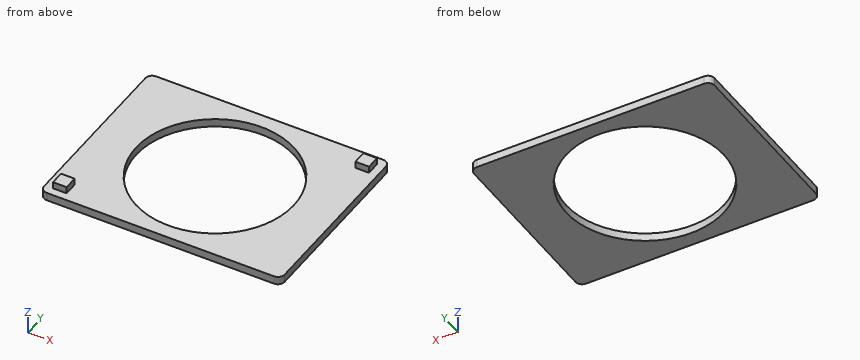
```python
from build123d import *

# Parameters (mm, degrees)
SKETCH007_W        = 35.4
SKETCH007_H        = 27.4
PAD002_DEPTH       = 1.2
FILLET001_R        = 1
SKETCH008_R        = 11.6
POCKET003_DEPTH    = 1.201
SKETCH009_W        = 2
SKETCH009_H        = 2
PAD003_DEPTH       = 1
POLARPATTERN_COUNT = 2


with BuildPart() as part:
    # Sketch007 → Pad002 (new body)
    with BuildSketch(Plane.XY):
        Rectangle(SKETCH007_W, SKETCH007_H)
    extrude(amount=PAD002_DEPTH)

    # Fillet001
    fillet001_edges = [part.edges().sort_by_distance(p)[0] for p in [
        (-17.7, -13.7, 0.6),
        (17.7, -13.7, 0.6),
        (17.7, 13.7, 0.6),
        (-17.7, 13.7, 0.6),
    ]]
    fillet(fillet001_edges, radius=FILLET001_R)

    # Sketch008 (on Face5 of Fillet001) → Pocket003 (cut, through all)
    with BuildSketch(Plane.XY.offset(1.2)):
        Circle(SKETCH008_R)
    extrude(amount=-POCKET003_DEPTH, mode=Mode.SUBTRACT)

    # Sketch009 (on Face5 of Pocket003) → Pad003 (join)
    with BuildSketch(Plane.XY.offset(1.2)):
        with Locations((-15.5, -11.5)):
            Rectangle(SKETCH009_W, SKETCH009_H)
    pad003 = extrude(amount=PAD003_DEPTH)

    # PolarPattern: Pad003 ×2 about axis
    polarpattern_axis = Axis((0, 0, 1.2), (0, 0, 1))
    for i in range(1, POLARPATTERN_COUNT):
        add(pad003.rotate(polarpattern_axis, i * 360 / POLARPATTERN_COUNT))


with BuildPart() as part_1:
    # Body002 placement: moved
    add(part.part.moved(Location((50, 0, 0))))


solid = part_1.part
```
For this review, take the finished solid that the model builds, in its own axes (mm). Coordinates: 2 decimals unless noted, no trailing zeros. Loops run counter-clockwise (first coordinate to the right, second up) from the corner with the lowest first, then second, coordinate; pieces in that order, holes last.
1. For line 1 (Y direction, x = 50, z = 0.3); line 2 (Z direction, x = 60, y = -6.5); line 3 (Y direction, x = 41, z = 0.7), list the stretches that pass through material, from the lowest coordinate up.
2. Insertion check: P1, Ø0.5, axis at y = -11, z = 2, coming from the -X side; P2, Ø0.8, axis at x = 65.5, z = 2, coming from the +Y side; P3, Ø0.5, axis at y = 11, z = 2, coming from the +X side. Each pin has a flat end and moves straight along its axis. Give the tip position at first contact, or say it passes through.
3. Add section B-B, the plane z = 1.75. Give the boundary of the cut face in (x, y), then the cut area to 3 significant figures.
4. Add section A-A, the plane x = 50. Give the boundary of the cut face in (y, z).
Result:
1. line 1: y = -13.7 to -11.6, 11.6 to 13.7
1. line 2: z = 0 to 1.2
1. line 3: y = -13.7 to -7.32, 7.32 to 13.7
2. P1: stops at x = 33.5
2. P2: stops at y = 12.5
2. P3: stops at x = 66.5
3. outline: (33.5, -12.5) - (35.5, -12.5) - (35.5, -10.5) - (33.5, -10.5) - close; (64.5, 10.5) - (66.5, 10.5) - (66.5, 12.5) - (64.5, 12.5) - close
3. area: 8.00 mm2
4. outline: (-13.7, 0) - (-11.6, 0) - (-11.6, 1.2) - (-13.7, 1.2) - close; (11.6, 0) - (13.7, 0) - (13.7, 1.2) - (11.6, 1.2) - close
